For this review, take the finished solid that the model builds, in its own axes (mm). Face numbers are marked on the shaded views. A direction names the side the tool comes from. Round coordinates to 2 decimals unless told otherwise and drop trailing zeros. Order: outer loops, then holes, each group sorted by start corner. A loop starts at its lowest first (then second) coordinate and runs counter-clockwise, first axis right, second up. Notation, with made-up numbers: M 50,-25.5 L 70,-25.5 A35 cw 70,9.5 Z; hole C 45,-29.75 d1. An arc over 180 degrees is marked long. Write item = value, one per line. Start each with the question number.
from build123d import *

# Parameters (mm, degrees)
BOSS_EXTRUDE1_DEPTH     = 33
CUT_EXTRUDE1_DEPTH      = 83.954293528
CUT_EXTRUDE1_DEPTH_BACK = 12
SKETCH3_W               = 9.481209811
SKETCH3_H               = 17.021727652
CUT_EXTRUDE2_DEPTH      = 22
SKETCH6_W               = 39.175540074
SKETCH6_H               = 11.416045591
BOSS_EXTRUDE3_DEPTH     = 26


with BuildPart() as part:
    # Sketch1 → Boss-Extrude1 (new body)
    with BuildSketch(Plane(origin=(0, 0, 0), x_dir=(1, 0, 0), z_dir=(0, 1, 0))):
        with BuildLine():
            Line((27.99701897, 26.104397373), (30.497019389, 26.104397373))
            Line((30.497019389, 26.104397373), (32.996926828, 26.125958592))
            Line((32.996926828, 26.125958592), (32.946330796, 31.992296402))
            ThreePointArc((32.946330796, 31.992296402), (34.614300355, 33.056919945), (35.86386473, 34.591238885))
            Line((35.86386473, 34.591238885), (40.431539769, 35.753760832))
            Line((40.431539769, 35.753760832), (43.136211097, 35.223788843))
            Line((43.136211097, 35.223788843), (43.274382132, 19.203600277))
            Line((43.274382132, 19.203600277), (48.774177579, 19.251034952))
            Line((48.774177579, 19.251034952), (48.43630867, 58.425118026))
            Line((48.43630867, 58.425118026), (42.936513223, 58.377683351))
            Line((42.936513223, 58.377683351), (43.088196039, 40.790876563))
            Line((43.088196039, 40.790876563), (40.395268448, 39.959225491))
            Line((40.395268448, 39.959225491), (35.888631414, 40.775372904))
            ThreePointArc((35.888631414, 40.775372904), (33.583892359, 43.097075019), (30.420151943, 43.929462788))
            ThreePointArc((30.420151943, 43.929462788), (27.263708108, 43.06982034), (24.979078258, 40.728327384))
            Line((24.979078258, 40.728327384), (20.479647685, 39.873342894))
            Line((20.479647685, 39.873342894), (17.779647685, 40.681737919))
            Line((17.779647685, 40.681737919), (17.779647685, 58.269198812))
            Line((17.779647685, 58.269198812), (12.279647685, 58.269198812))
            Line((12.279647685, 58.269198812), (12.279647685, 19.093658738))
            Line((12.279647685, 19.093658738), (17.779647685, 19.093658738))
            Line((17.779647685, 19.093658738), (17.779647685, 35.114443143))
            Line((17.779647685, 35.114443143), (20.479647685, 35.667721822))
            Line((20.479647685, 35.667721822), (25.057179, 34.544636961))
            ThreePointArc((25.057179, 34.544636961), (26.319929615, 33.021151936), (27.99701897, 31.970953369))
            Line((27.99701897, 31.970953369), (27.99701897, 26.104397373))
        make_face()
    extrude(amount=BOSS_EXTRUDE1_DEPTH)

    # Sketch2 → Cut-Extrude1 (cut, two sides: drawn at the far end of the back side and taken through both)
    with BuildSketch(Plane.XZ.offset(-CUT_EXTRUDE1_DEPTH_BACK)):
        with BuildLine():
            Line((20.479647685, -35.667721822), (17.779647685, -35.114443143))
            Line((17.779647685, -35.114443143), (17.779647685, -40.681737919))
            Line((17.779647685, -40.681737919), (20.479647685, -39.873342894))
            Line((20.479647685, -39.873342894), (24.979078258, -40.728327384))
            ThreePointArc((24.979078258, -40.728327384), (27.263708108, -43.06982034), (30.420151943, -43.929462788))
            ThreePointArc((30.420151943, -43.929462788), (33.576595778, -43.084424394), (35.888631414, -40.775372904))
            Line((35.888631414, -40.775372904), (40.395268448, -39.959225491))
            Line((40.395268448, -39.959225491), (43.088196039, -40.790876563))
            Line((43.088196039, -40.790876563), (43.136211097, -35.223788843))
            Line((43.136211097, -35.223788843), (40.431539769, -35.753760832))
            Line((40.431539769, -35.753760832), (35.86386473, -34.591238885))
            ThreePointArc((35.86386473, -34.591238885), (34.614300355, -33.056919945), (32.946330796, -31.992296402))
            Line((32.946330796, -31.992296402), (32.996926828, -26.125958592))
            Line((32.996926828, -26.125958592), (27.99701897, -26.104397373))
            Line((27.99701897, -26.104397373), (27.99701897, -31.970953369))
            ThreePointArc((27.99701897, -31.970953369), (26.319929615, -33.021151936), (25.057179, -34.544636961))
            Line((25.057179, -34.544636961), (20.479647685, -35.667721822))
        make_face()
    extrude(amount=CUT_EXTRUDE1_DEPTH + CUT_EXTRUDE1_DEPTH_BACK, mode=Mode.SUBTRACT)

    # Sketch3 → Cut-Extrude2 (cut)
    with BuildSketch(Plane.XY.offset(-26.104397373)):
        with Locations((32.737623876, 3.489136174)):
            Rectangle(SKETCH3_W, SKETCH3_H)
    extrude(amount=-CUT_EXTRUDE2_DEPTH, mode=Mode.SUBTRACT)

    # Sketch6 → Boss-Extrude3 (add)
    with BuildSketch(Plane(origin=(17.779647685, 0, 0), x_dir=(0, 0, -1), z_dir=(1, 0, 0))):
        with Locations((38.681428775, 27.291977205)):
            Rectangle(SKETCH6_W, SKETCH6_H)
    extrude(amount=BOSS_EXTRUDE3_DEPTH)


solid = part.part
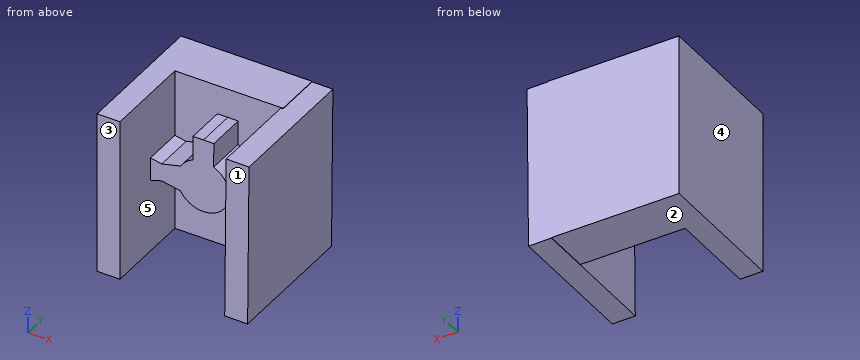
(1) For line 1 along Z through (x, y) = (47.5, 12); line 2 along Y through (x, z) = (42, -24); line 3 along Y through (x, z) = (33.5, -42.5), list the stretches that pass through material, from the lowest coordinate up.
(2) Insertion check: pin 1 (4 mm diameter, centred on x = 30.5, y = 13, fed in from +Z); pin 2 (12 mm diameter, centred on x = 32, z = -40.5, fed in from -Y); pin 3 (10 mm diameter, centred on x = 32, y = 19.5, fed in from -Z); pin 4 (3 mm diameter, centred on x = 20, y = 3.5, fed in from +Z). Each pin has a flat end and moves straight along its axis. Give the tip position at first contact, or say it passes through.
(3) We need section C-C, the plane x = 41. Write out the cut boundary in (y, z), then the cut area to 3 significant figures.
(4) We need section A-A, the plane y = 4.5. Write out the cut boundary in (x, z).
(5) For the marked faces 1 and 2, list the 3-axis set-ups (+Z, -Z, +X, -X, +Y, -Y) from which the entire face can be reached by the end or side of a thin tool; tool diameter is ignored.
(6) We need section B-B, the plane y = 16.5. Write out the cut boundary in (x, z), then the cut area to 3 significant figures.
(7) Draft analysis for pull direction X (two halves, no side actions). For the marked faces 3, 4 and 5, state which applies: released by +X, released by -X, zero draft, split by the parting line, or undercut.
(8) We need section D-D, the plane z = -30.5. Write out the cut boundary in (x, y).
Values:
q1.line_1 = -58.42 to -19.24
q1.line_2 = 21.58 to 33
q1.line_3 = 12 to 33
q2.pin_1 = -26.1
q2.pin_2 = 12
q2.pin_3 = -58.27
q2.pin_4 = through
q3.outline = M 12,-40.15 L 21.58,-40.15 L 21.58,-58.27 L 33,-58.27 L 33,-19.09 L 21.58,-19.09 L 21.58,-35.64 L 12,-35.64 Z
q3.area = 490 mm²
q4.outline = M 12.28,-58.27 L 17.78,-58.27 L 17.78,-19.09 L 12.28,-19.09 Z; M 42.94,-58.38 L 48.44,-58.43 L 48.77,-19.25 L 43.27,-19.2 Z
q5.face_1 = +Z, -Z, +X, -X, -Y
q5.face_2 = -Z, -X, +Y, -Y
q6.outline = M 12.28,-58.27 L 17.78,-58.27 L 17.78,-40.68 L 20.48,-39.87 L 24.98,-40.73 A6.22 ccw 30.42,-43.93 A6.22 ccw 35.89,-40.78 L 40.4,-39.96 L 43.09,-40.79 L 42.94,-58.38 L 48.44,-58.43 L 48.77,-19.25 L 43.27,-19.2 L 43.14,-35.22 L 40.43,-35.75 L 35.86,-34.59 A6.22 ccw 32.95,-31.99 L 33,-26.13 L 30.5,-26.1 L 28,-26.1 L 28,-31.97 A6.22 ccw 25.06,-34.54 L 20.48,-35.67 L 17.78,-35.11 L 17.78,-19.09 L 12.28,-19.09 Z
q6.area = 648 mm²
q7.face_3 = zero draft
q7.face_4 = released by -X
q7.face_5 = undercut
q8.outline = M 12.28,0 L 17.78,0 L 17.78,21.58 L 28,21.58 L 28,12 L 32.96,12 L 32.96,21.58 L 43.18,21.58 L 43.18,0 L 48.68,0 L 48.68,33 L 12.28,33 Z
